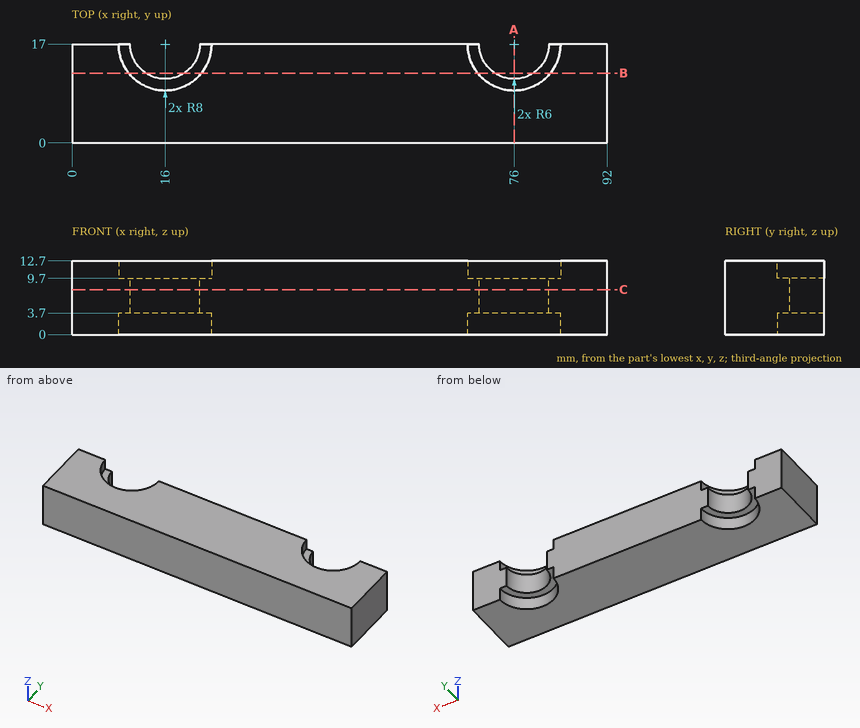
Geometry check sheet. Reference: drawing and pictorial views, mm from the part's lowest x, y, z. Give positions to 0.01 mm unless a question says otherwise; leave off trailing zeros. Order: outer loops, then holes, each group sorted by start corner. A loop starts at its lowest first (then second) coordinate and runs counter-clockwise, first axis right, second up. Notation, with made-up numbers: (66.5, 74.5) -> (90.5, 74.5) arc R12 ccw to (90.5, 84.5) -> close; hole circle Ø9 at (2, -32). An arc over 180 degrees is marked (long way). Write each question's results on one line, items separated by ' | '. Start each with the question number.
(1) Sectioned sample at C-C (z = 7.75). Enter the section's corners in (x, y), plus the area to 3 significant figures.
(2) Sectioned sample at A-A (x = 76). Enter the section's corners in (y, z), plus the area to 3 significant figures.
(3) Scan lines: line 1 (X direction, y = 15.25, z = 10.5); line 2 (X direction, y = 10.25, z = 10.75); line 3 (Z direction, x = 12, y = 12). Record each from-to range of solid material in increasing order.
(4) Sectioned sample at B-B (y = 12). Enter the section's corners in (x, z) (3 decimals).
Answer below:
1) outline: (0, 0) -> (92, 0) -> (92, 17) -> (82, 17) arc R6 cw to (70, 17) -> (22, 17) arc R6 cw to (10, 17) -> (0, 17) -> close | area: 1,450 mm2
2) outline: (0, 0) -> (9, 0) -> (9, 3.7) -> (11, 3.7) -> (11, 9.7) -> (9, 9.7) -> (9, 12.7) -> (0, 12.7) -> close | area: 126 mm2
3) line 1: 0 to 8.19, 23.81 to 68.19, 83.81 to 92 | line 2: 0 to 11.71, 20.29 to 71.71, 80.29 to 92 | line 3: 3.7 to 9.7
4) outline: (0, 0) -> (9.755, 0) -> (9.755, 3.7) -> (12.683, 3.7) -> (12.683, 9.7) -> (9.755, 9.7) -> (9.755, 12.7) -> (0, 12.7) -> close; (19.317, 3.7) -> (22.245, 3.7) -> (22.245, 0) -> (69.755, 0) -> (69.755, 3.7) -> (72.683, 3.7) -> (72.683, 9.7) -> (69.755, 9.7) -> (69.755, 12.7) -> (22.245, 12.7) -> (22.245, 9.7) -> (19.317, 9.7) -> close; (79.317, 3.7) -> (82.245, 3.7) -> (82.245, 0) -> (92, 0) -> (92, 12.7) -> (82.245, 12.7) -> (82.245, 9.7) -> (79.317, 9.7) -> close
